Verification items for the finished model (mm, model axes). A direction names the side the tool comes from. Round coordinates to 2 decimals unless told otherwise and drop trailing zeros. Write each loop counter-clockwise with the first axis right and the second up, starting at its lowest first coordinate (ties: lowest second). Pieces come first, ordered by that corner, then holes. Notation, with made-up numbers: (0, -4.75) -> (8, -4.75) arc R29 ccw to (8, 28.25) -> close; hole circle Ø11 at (-19, 48). An arc over 180 degrees is marked (long way). Answer as a JSON object with one key per item and string values. Group by question number.
(1) Sectioned sample at D-D on y = 3.75. Record the cut outline in (x, z).
(2) Scan lines: L1, parallel to Y at x = -3.85, z = 57.5; L2, parallel to Z at x = -5.65, y = 0; L3, parallel to Z at x = 0.05, y = 0. Record each from-to range of solid material in increasing order. Write a range as from..to.
(3) Set-up check for faces 1 (the face through (4, 5, 54)), 2 (the face through (2.5, -0.1, -4.8)), 3 (the face through (-2.5, -0.1, 54.8)), 4 (the face through (0, 5, -4)): record each of +Z, -Z, +X, -X, +Y, -Y from which the full face is reachable in a straight line by a thin tool's end or side.
(4) Sectioned sample at A-A on x = 0. Record the cut outline in (y, z), and give its area (3 significant figures).
(5) Sectioned sample at C-C on z = -2.5. Record the cut outline in (x, y).
(6) Draft check along X on faces 5 (the face through (-2.5, -0.1, -4.8)), 6 (the face through (2.5, -0.1, 54.8)), 7 (the face through (0, -5, -4)). Enter one of: released by +X, released by -X, zero draft, split by the parting line, or undercut.
(7) Sectioned sample at B-B on y = 1. Record the cut outline in (x, z).
(8) Gauge pin test, flat ends, axial feed: pin 1 Ø5 at (x, y) = (0, -2.5) entering from -Z; pin 2 Ø2 at (x, z) = (-3, 36) entering from -Y; pin 3 Ø3 at (y, z) = (4, 53.5) entering from -X; pin 4 Ø8 at (y, z) = (0, -7.5) entering from +X. Record the tip position at first contact, or that the pin passes through.
```python
from build123d import *

# Parameters (mm, degrees)
CROQUIS1_R                   = 7.5
SALIENTE_EXTRUIR1_DEPTH      = 50
CROQUIS4_W                   = 5
CROQUIS4_H                   = 10
SALIENTE_EXTRUIR2_DEPTH      = 12.5
CROQUIS5_R                   = 2.5
CORTAR_EXTRUIR1_DEPTH        = 5
SALIENTE_EXTRUIR4_DEPTH      = 7.5
SALIENTE_EXTRUIR4_DEPTH_BACK = 7.5
CROQUIS9_R                   = 2.5
CROQUIS10_W                  = 5
CROQUIS10_H                  = 10
CORTAR_EXTRUIR2_DEPTH        = 12.5
CROQUIS11_R                  = 10
CROQUIS11_R_2                = 7.5
CORTAR_EXTRUIR3_DEPTH        = 12.5


with BuildPart() as part:
    # Croquis1 → Saliente-Extruir1 (new body)
    with BuildSketch(Plane.XY):
        Circle(CROQUIS1_R)
    extrude(amount=SALIENTE_EXTRUIR1_DEPTH)

    # Croquis4 → Saliente-Extruir2 (add)
    with BuildSketch(Plane(origin=(0, 0, 0), x_dir=(-1, 0, 0), z_dir=(0, 0, -1))):
        Rectangle(CROQUIS4_W, CROQUIS4_H)
    extrude(amount=SALIENTE_EXTRUIR2_DEPTH)

    # Croquis5 → Cortar-Extruir1 (cut)
    with BuildSketch(Plane.ZY.offset(2.5)):
        with BuildLine():
            ThreePointArc((-7.5, -5), (-11.035533906, -3.535533906), (-12.5, 0))
            Line((-12.5, 0), (-12.5, -5))
            Line((-12.5, -5), (-7.5, -5))
        make_face()
        with BuildLine():
            ThreePointArc((-12.5, 0), (-11.035533906, 3.535533906), (-7.5, 5))
            Line((-7.5, 5), (-12.5, 5))
            Line((-12.5, 5), (-12.5, 0))
        make_face()
        with Locations(Location((-7.5, 0, 0), (0, 0, 270))):
            Circle(CROQUIS5_R)
    extrude(amount=-CORTAR_EXTRUIR1_DEPTH, mode=Mode.SUBTRACT)

    # Croquis9 → Saliente-Extruir4 (add, two sides: drawn at the far end of the back side and taken through both)
    with BuildSketch(Plane(origin=(0, 0, 0), x_dir=(0, 0, -1), z_dir=(1, 0, 0)).offset(-SALIENTE_EXTRUIR4_DEPTH_BACK)):
        with BuildLine():
            Line((-50, -5), (-50, 5))
            Line((-50, 5), (-57.5, 5))
            ThreePointArc((-57.5, 5), (-61.035533906, 3.535533906), (-62.5, 0))
            ThreePointArc((-62.5, 0), (-61.035533906, -3.535533906), (-57.5, -5))
            Line((-57.5, -5), (-50, -5))
        make_face()
        with Locations((-57.5, 0)):
            Circle(CROQUIS9_R, mode=Mode.SUBTRACT)
    extrude(amount=SALIENTE_EXTRUIR4_DEPTH + SALIENTE_EXTRUIR4_DEPTH_BACK)

    # Croquis10 → Cortar-Extruir2 (cut)
    with BuildSketch(Plane.XY.offset(50)):
        Rectangle(CROQUIS10_W, CROQUIS10_H)
    extrude(amount=CORTAR_EXTRUIR2_DEPTH, mode=Mode.SUBTRACT)

    # Croquis11 → Cortar-Extruir3 (cut)
    with BuildSketch(Plane.XY.offset(50)):
        Circle(CROQUIS11_R)
        with Locations(Location((0, 0, 0), (0, 0, 221.810314896))):
            Circle(CROQUIS11_R_2, mode=Mode.SUBTRACT)
    extrude(amount=CORTAR_EXTRUIR3_DEPTH, mode=Mode.SUBTRACT)


solid = part.part
```
Computed values:
{
 "1": {"outline": "(-6.5, 0) -> (-2.5, 0) -> (-2.5, -10.81) -> (2.5, -10.81) -> (2.5, 0) -> (6.5, 0) -> (6.5, 60.81) -> (2.5, 60.81) -> (2.5, 50) -> (-2.5, 50) -> (-2.5, 60.81) -> (-6.5, 60.81) -> close"},
 "2": {"L1": "-5..-2.5, 2.5..5", "L2": "0..55, 60..62.5", "L3": "-12.5..-10, -5..50"},
 "3": {"face 1": "+Z, +X, -X, +Y", "face 2": "-Z, +X, +Y, -Y", "face 3": "+Z, +Y, -Y", "face 4": "-Z, +X, -X, +Y"},
 "4": {"outline": "(-7.5, 0) -> (-5, 0) -> (-5, -7.5) arc R5 ccw to (5, -7.5) -> (5, 0) -> (7.5, 0) -> (7.5, 50) -> (-7.5, 50) -> close; hole circle Ø5 at (0, -7.5)", "area": "845 mm2"},
 "5": {"outline": "(-2.5, -5) -> (2.5, -5) -> (2.5, 5) -> (-2.5, 5) -> close"},
 "6": {"face 5": "released by -X", "face 6": "undercut", "face 7": "zero draft"},
 "7": {"outline": "(-7.43, 0) -> (-2.5, 0) -> (-2.5, -5.21) -> (2.5, -5.21) -> (2.5, 0) -> (7.43, 0) -> (7.43, 55.21) -> (2.5, 55.21) -> (2.5, 50) -> (-2.5, 50) -> (-2.5, 55.21) -> (-7.43, 55.21) -> close; (-7.43, 59.79) -> (-2.5, 59.79) -> (-2.5, 62.4) -> (-7.43, 62.4) -> close; (-2.5, -12.4) -> (2.5, -12.4) -> (2.5, -9.79) -> (-2.5, -9.79) -> close; (2.5, 59.79) -> (7.43, 59.79) -> (7.43, 62.4) -> (2.5, 62.4) -> close"},
 "8": {"pin 1": "z = -12.5", "pin 2": "y = -7.23", "pin 3": "x = -7.07", "pin 4": "x = 2.5"}
}
